Autodesk Fusion 360 part; units mm, degrees
sketch "Sketch1" plane through (0, 0, 0) normal (0, 0, 1) x (1, 0, 0)
  circle A0 centre (0, 0) radius 2.5
  dimension "d1" = 5
extrude "Extrude1" add sketch "Sketch1" along normal blind 20
fillet "Fillet1" radius 0.1 1 edges at (-2.3308, -0.904, 0)
fillet "Fillet2" radius 0.1 1 edges at (-2.3308, -0.904, 20)
sketch "Sketch2" plane through (0, 0, 20) normal (0, 0, 1) x (-1, 0, 0)
  circle A0 centre (0, 0) radius 2.4
  circle A1 centre (0, 0) radius 2.25
  dimension "d8" = 4.5
extrude "Extrude2" cut sketch "Sketch2" against normal blind 0.2 contours A1
fillet "Fillet3" radius 0.1 1 edges at (2.0977, -0.8136, 20)
sketch "Sketch3" plane through (0, 0, 19.8) normal (0, 0, 1) x (-1, 0, 0)
  circle A0 centre (0, 0) radius 2.25
  circle A1 centre (0, 0) radius 1
  dimension "d13" = 2
extrude "Extrude3" add sketch "Sketch3" along normal blind 0.5 contours A1
fillet "Fillet4" radius 0.1 1 edges at (0.9323, 0.3616, 20.3)
Design review of the part built by this model. Coordinates are the model's own, in mm. A direction names the side the tool comes from. Round coordinates to 2 decimals unless told otherwise and drop trailing zeros. Write each loop counter-clockwise with the first axis right and the second up, starting at its lowest first coordinate (ties: lowest second). Pieces come first, ordered by that corner, then holes. Notation, with made-up numbers: (15, 26) - (46, 26) arc R16 ccw to (46, 33) - close; hole circle Ø6 at (36.5, 56.25). An arc over 180 degrees is marked (long way). Return JSON: item names as keys, results as strings. Group by question number.
Item 1: Insertion check: P1, Ø3, axis at x = 1.5, y = -1.5, coming from the +Z side; P2, Ø1, axis at y = 1, z = 8, coming from the +X side; P3, Ø1.5, axis at x = 1, z = 8, coming from the +Y side. Each pin has a flat end and moves straight along its axis. Give the tip position at first contact, or say it passes through.
Item 2: For probe 1 along Y at (x, z) = (0, 19.9); probe 2 along Z at (x, y) = (1.6, 0.3); probe 3 along X at (y, z) = (0.1, 10), list the stretches that pass through material, from the lowest coordinate up. Write a range as [from, to].
Item 3: We need section A-A on z = 7. Write out the cut boundary in (x, y).
Item 4: Machinability: for faces 1 (the face through (0, 0, 20.3)), 2 (the face through (1, 1, 19.8)), which of the approach directions +Z, -Z, +X, -X, +Y, -Y give a long, thin tool a straight path to every point of the face, cutting with its end or side? Answer none if there is none.
Item 5: The part is to be moulded in two halves that separate along X. For faces 3 (the face through (0, -1, 20)), 4 (the face through (0, 0, 0)), 5 (the face through (-0.54, 2.44, 9.86)), say which applies: pulls with the +X half, pulls with the -X half, needs draft (parallel to the pull), parting line crosses it, or undercut.
Model answer:
{
 "1": {"P1": "stops at z = 20.3", "P2": "stops at x = 2.45", "P3": "stops at y = 2.49"},
 "2": {"probe 1": "y = [-2.5, -2.25], [-1, 1], [2.25, 2.5]", "probe 2": "z = [0, 19.8]", "probe 3": "x = [-2.5, 2.5]"},
 "3": {"outline": "circle Ø5 at (0, 0)"},
 "4": {"face 1": "+Z, +X, -X, +Y, -Y", "face 2": "+Z"},
 "5": {"face 3": "undercut", "face 4": "needs draft", "face 5": "parting line crosses it"}
}
